Model file for the job. Use its own axes, mm. A direction names the side the tool comes from. Coordinates: 2 decimals unless noted, no trailing zeros. Order: outer loops, then holes, each group sorted by start corner. A loop starts at its lowest first (then second) coordinate and runs counter-clockwise, first axis right, second up. Notation, with made-up numbers: (-1, 75.5) -> (26, 75.5) arc R10 cw to (26, 93.5) -> close; hole circle Ø8 at (-12, -26). An arc over 180 degrees is marked (long way). Write item = value, one per line. Start each with the question number.
Q1. Cut at B-B, the plane x = 183. List the corners of the cut face in (y, z), plus the area to 4 significant figures.
Q2. Cut at C-C, the plane y = -23. List the corners of the cut face in (x, z).
Q3. 3-axis set-ups, long thin cutter, end or side, ignore diameter. For faces 1 (the face through (225, 0, 1)), 2 (the face through (-3, 0, 1.5)), 3 (the face through (-3, 0, 0)): which of +Z, -Z, +X, -X, +Y, -Y reach the whole face in a straight line?
Q4. Flat gauge pins, fed straight in: pin 1 (2 mm diameter, centred on x = -75, y = -21, fed in from +Z); pin 2 (5 mm diameter, centred on y = -29.5, z = -1.5, fed in from -X); pin 3 (1 mm diameter, centred on x = -69, y = 0.5, fed in from -Z). Where does each tip first touch, or does it go through?
Q5. Wall check: line 1 (Y direction, x = 173, z = 2.5); line 2 (Z direction, x = 65.5, y = 14.5). Give the ranges that are in metal, low to high. Write a range as from..to.
Q6. Cut at A-A, the plane z = 5.75. List the corners of the cut face in (x, y), plus the area to 3 significant figures.
from build123d import *

# Parameters (mm, degrees)
F0_W     = 450
F0_H     = 75
F1_DEPTH = 1.5
F2_W     = 450
F2_H     = 6.5
F3_DEPTH = 6.5
F4_W     = 450
F4_H     = 6.5
F5_DEPTH = 6.5


with BuildPart() as f1:
    # F0 (on Top) → F1 (new body)
    with BuildSketch(Plane.XY):
        Rectangle(F0_W, F0_H)
    extrude(amount=F1_DEPTH)

    # F2 (on face) → F3 (join)
    with BuildSketch(Plane.XY.offset(1.5)):
        with Locations((0, -34.25)):
            Rectangle(F2_W, F2_H)
        with Locations((0, 34.25)):
            Rectangle(F2_W, F2_H)
    extrude(amount=F3_DEPTH)

    # F4 (on face) → F5 (join)
    with BuildSketch(Plane(origin=(0, 0, 0), x_dir=(1, 0, 0), z_dir=(0, 0, -1))):
        with Locations((0, 34.25)):
            Rectangle(F4_W, F4_H)
        with Locations((0, -34.25)):
            Rectangle(F4_W, F4_H)
    extrude(amount=F5_DEPTH)


solid = f1.part
Here are the results:
q1.outline = (-37.5, -6.5) -> (-31, -6.5) -> (-31, 0) -> (31, 0) -> (31, -6.5) -> (37.5, -6.5) -> (37.5, 8) -> (31, 8) -> (31, 1.5) -> (-31, 1.5) -> (-31, 8) -> (-37.5, 8) -> close
q1.area = 281.5 mm²
q2.outline = (-225, 0) -> (225, 0) -> (225, 1.5) -> (-225, 1.5) -> close
q3.face_1 = +Z, -Z, +X, +Y, -Y
q3.face_2 = +Z, +X, -X
q3.face_3 = -Z, +X, -X
q4.pin_1 = 1.5
q4.pin_2 = -225
q4.pin_3 = 0
q5.line_1 = -37.5..-31, 31..37.5
q5.line_2 = 0..1.5
q6.outline = (-225, -37.5) -> (225, -37.5) -> (225, -31) -> (-225, -31) -> close; (-225, 31) -> (225, 31) -> (225, 37.5) -> (-225, 37.5) -> close
q6.area = 5,850 mm²
